Verification items for the finished model (mm, model axes). Face numbers are marked on the shaded views. Give positions to 0.01 mm unless a question says otherwise; leave off trailing zeros. Order: outer loops, then holes, each group sorted by start corner. A loop starts at its lowest first (then second) coordinate and runs counter-clockwise, first axis right, second up. Notation, with made-up numbers: (61.5, 54.5) -> (108.5, 54.5) arc R19 ccw to (108.5, 66.5) -> close; hole circle Ø6 at (-39, -24.5). An arc over 180 degrees is marked (long way). Return JSON: item names as keys, results as strings. Group by question number.
(1) Cross-section at B-B on z = 122. Enter the section's corners in (x, y).
(2) Thickness scan on line 1 along Z through (x, y) = (12.7, 0.5); line 2 along X through (y, z) = (2, 129.5); line 3 along X through (y, z) = (2.3, 109.5). Record the ranges inside material, lowest first.
(3) Release check for a two-part mould opening along Y. For the marked faces 1 and 2 record: pulls with the +Y half, pulls with the -Y half, needs draft (parallel to the pull), parting line crosses it, or undercut.
(4) Cross-section at A-A on y = 1.1. State how many separate pieces and enclosed holes the cut face has, then the cut area to 3 significant figures.
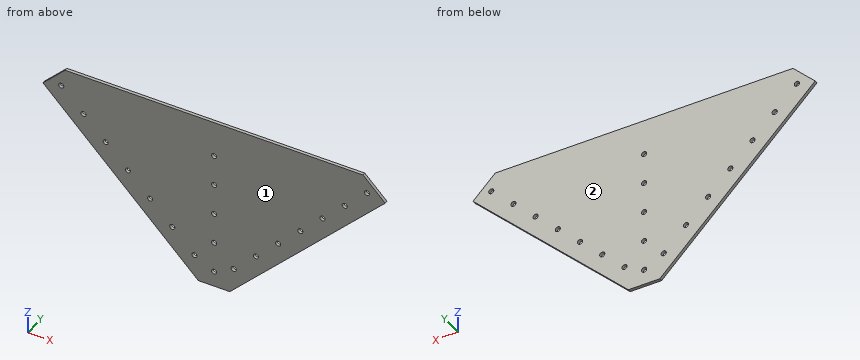
from build123d import *

# Parameters (mm, degrees)
BOSS_EXTRUDE1_DEPTH        = 2.54
CUT_EXTRUDE1_DEPTH         = 209.542345228
CUT_EXTRUDE1_DEPTH_BACK    = 209.542345228
SKETCH2_R                  = 2.0955
F_8_0_199_DIAMETER_HOLE1_D = 4.191


with BuildPart() as part:
    # Sketch1 → Boss-Extrude1 (new body)
    with BuildSketch(Plane(origin=(0, 0, 0), x_dir=(1, 0, 0), z_dir=(0, 1, 0))):
        Polygon((0, 0), (25.4, 0), (151.123585695, -125.723585695), (133.163073453, -143.684097937), (-107.763073453, -143.684097937), (-125.723585695, -125.723585695), align=None)
    extrude(amount=BOSS_EXTRUDE1_DEPTH)

    # Sketch2 → Cut-Extrude1 (cut, two sides: drawn at the far end of the back side and taken through both)
    with BuildSketch(Plane(origin=(0, 2.54, 0), x_dir=(1, 0, 0), z_dir=(0, 1, 0)).offset(-CUT_EXTRUDE1_DEPTH_BACK)):
        with Locations(Location((12.7, -12.7, 0), (0, 0, 270))):
            Circle(SKETCH2_R)
        with Locations(Location((12.7, -38.1, 0), (0, 0, 270))):
            Circle(SKETCH2_R)
        with Locations(Location((12.7, -63.5, 0), (0, 0, 270))):
            Circle(SKETCH2_R)
        with Locations(Location((12.7, -88.9, 0), (0, 0, 270))):
            Circle(SKETCH2_R)
        with Locations(Location((12.7, -114.3, 0), (0, 0, 270))):
            Circle(SKETCH2_R)
    extrude(amount=CUT_EXTRUDE1_DEPTH + CUT_EXTRUDE1_DEPTH_BACK, mode=Mode.SUBTRACT)

    # #8 (0.199) Diameter Hole1 (through all)
    with Locations(Plane(origin=(0, 0, 0), x_dir=(-1, 0, 0), z_dir=(0, -1, 0))):
        with Locations((21.151548005, -39.112060247), (39.112060247, -57.072572489), (57.072572489, -75.033084731), (75.033084731, -92.993596973), (92.993596973, -110.954109215), (110.954109215, -128.914621458), (-28.591035763, -21.151548005), (-46.551548005, -39.112060247), (-64.512060247, -57.072572489), (-82.472572489, -75.033084731), (-100.433084731, -92.993596973), (-118.393596973, -110.954109215), (-136.354109215, -128.914621458), (3.191035763, -21.151548005)):
            Hole(F_8_0_199_DIAMETER_HOLE1_D / 2)


solid = part.part
Verdict:
{
 "1": {"outline": "(-122, 0) -> (147.4, 0) -> (147.4, 2.54) -> (-122, 2.54) -> close"},
 "2": {"line 1": "0 to 10.6, 14.8 to 36, 40.2 to 61.4, 65.6 to 86.8, 91 to 112.2, 116.4 to 143.68", "line 2": "-121.95 to -112.97, -108.94 to 134.34, 138.37 to 147.35", "line 3": "-109.5 to -94.5, -91.48 to 116.88, 119.9 to 134.9"},
 "3": {"face 1": "pulls with the -Y half", "face 2": "pulls with the +Y half"},
 "4": {"separate pieces": "1", "enclosed holes": "19", "area": "23,400 mm²"}
}
